Build history of the part. All positions in model axes, mm. A direction names the side the tool comes from. Round coordinates to 2 decimals unless told otherwise and drop trailing zeros. Write each loop counter-clockwise with the first axis right and the second up, starting at its lowest first coordinate (ties: lowest second). Pieces come first, ordered by that corner, then holes. Notation, with made-up numbers: (14.25, 0.5) - (29.25, 0.5) arc R19 ccw to (29.25, 17.5) - close; hole circle Ø10 at (46, -12). An arc over 180 degrees is marked (long way). Answer as a JSON object with one key per item and string values. Group by question number.
Item 1: Flat gauge pins, fed straight in: pin 1 (2 mm diameter, centred on y = 4, z = -1, fed in from -X); pin 2 (3.5 mm diameter, centred on x = 0, y = 0, fed in from +Z); pin 3 (2 mm diameter, centred on x = -4.5, y = 3, fed in from -Z). Where does each tip first touch, or does it go through?
Item 2: Probe line 1 (Y direction, x = 0, z = 0.8); line 2 (Z direction, x = -1, y = 0.75); line 3 (X direction, y = 3.75, z = 1.15). List the from-to ranges inside material, lowest first. Write a range as from..to.
Item 3: Which spindle directions (+Z, -Z, +X, -X, +Y, -Y) get a long thin tool onto all of the face, cutting with end or side? Do faces 1 (the flat face through (3, 4, 0)), 2 (the cylindrical face through (-5.994, -0.264, -0.246)). Say none if no direction does.
Item 4: Slice it at C-C, the plane z = -2.25. List the corners of the cut face in (x, y), then the cut area to 3 significant figures.
Item 5: Slice it at D-D, the plane z = 1.4. List the corners of the cut face in (x, y).
Item 6: Slice it at A-A, the plane y = 0. List the corners of the cut face in (x, z), then the cut area to 4 significant figures.
from build123d import *

# Parameters (mm, degrees)
SKETCH_R     = 4.1
SKETCH_R_2   = 3.05
PAD_DEPTH    = 3
SKETCH001_R  = 6
PAD001_DEPTH = 3
CHAMFER_SIZE = 2.5


with BuildPart() as part:
    # Sketch → Pad (new body)
    with BuildSketch(Plane.XY):
        Circle(SKETCH_R)
        Circle(SKETCH_R_2, mode=Mode.SUBTRACT)
    extrude(amount=PAD_DEPTH)

    # Sketch001 (on Face3 of Pad) → Pad001 (join)
    with BuildSketch(Plane(origin=(0, 0, 0), x_dir=(1, 0, 0), z_dir=(0, 0, -1))):
        Circle(SKETCH001_R)
    extrude(amount=PAD001_DEPTH)

    # Chamfer
    chamfer_edges = [part.edges().sort_by_distance(p)[0] for p in [
        (-6, 0, -3),
    ]]
    chamfer(chamfer_edges, length=CHAMFER_SIZE)


solid = part.part
Geometry says:
{
 "1": {"pin 1": "stops at x = -5.12", "pin 2": "stops at z = 0", "pin 3": "stops at z = -2.09"},
 "2": {"line 1": "y = -4.1..-3.05, 3.05..4.1", "line 2": "z = -3..0", "line 3": "x = -1.66..1.66"},
 "3": {"face 1": "+Z", "face 2": "+Z, -Z"},
 "4": {"outline": "circle Ø8.5 at (0, 0)", "area": "56.7 mm^2"},
 "5": {"outline": "circle Ø8.2 at (0, 0); hole circle Ø6.1 at (0, 0)"},
 "6": {"outline": "(-6, -0.5) - (-3.5, -3) - (3.5, -3) - (6, -0.5) - (6, 0) - (4.1, 0) - (4.1, 3) - (3.05, 3) - (3.05, 0) - (-3.05, 0) - (-3.05, 3) - (-4.1, 3) - (-4.1, 0) - (-6, 0) - close", "area": "36.05 mm^2"}
}
